from build123d import *

# Parameters (mm, degrees)
F1_DEPTH = 34.925
F2_DEPTH = 11.1125
F3_SIZE2 = 11.11249
F3_SIZE  = 4.602938


# Not quite as in the source:
# - a fillet or chamfer is up to 0.001 mm smaller than in the source, because OpenCascade refuses the exact size


with BuildPart() as f1:
    # F0 (on Top) → F1 (new body)
    with BuildSketch(Plane.XY):
        Polygon((0, -134.14375), (0, 134.14375), (-73.81875, 0), align=None)
        Polygon((73.81875, 0), (0, 134.14375), (0, -134.14375), align=None)
    extrude(amount=-F1_DEPTH)

    # F0 (on Top) + F1_face (on face) → F2 (join)
    with BuildSketch(Plane.XY):
        Polygon((-103.1875, 0), (0, -187.5127688172), (103.1875, 0), (0, 187.5127688172), align=None)
        Polygon((-73.81875, 0), (0, 134.14375), (73.81875, 0), (0, -134.14375), align=None, mode=Mode.SUBTRACT)
    with BuildSketch(Plane.XY):
        Polygon((0, 134.14375), (-73.81875, 0), (0, -134.14375), (73.81875, 0), align=None)
    extrude(amount=F2_DEPTH)

    # F3 (size 4.6029482119 and 11.1125 in the source; OpenCascade refuses exactly that, so slightly less here)
    f3_edges = [f1.edges().sort_by_distance(p)[0] for p in [
        (-51.59375, -93.756384, 11.1125),
        (-51.59375, 93.756384, 11.1125),
        (51.59375, 93.756384, 11.1125),
        (51.59375, -93.756384, 11.1125),
    ]]
    f3_side = f1.faces().sort_by_distance((0, 0, 11.1125))[0]
    chamfer(f3_edges, length=F3_SIZE, length2=F3_SIZE2, reference=f3_side)


solid = f1.part
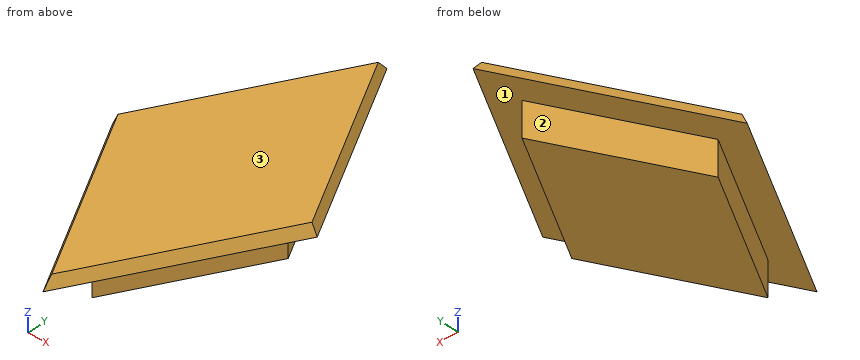
Input: part model. Units: mm. Frame: model coordinates. Face numbers are marked on the shaded views. A direction names the side the tool comes from. Give positions to 0.01 mm unless a question says otherwise; leave off trailing zeros. Order: outer loops, then holes, each group sorted by start corner. A loop starts at its lowest first (then second) coordinate and runs counter-clockwise, first axis right, second up.
Q1. Section C-C on z = -16. Output: boundary loops of the cut face in (x, y).
Checked values:
outline: (-73.82, 0) - (0, -134.14) - (73.82, 0) - (0, 134.14) - close
Q2. Ray query, probe 1 along X at (y, z) = (-92.5, 2.5); probe 2 along Y at (x, z) = (28, -25.5); probe 3 along X at (y, z) = (101.5, -11). Return the intervals inside material, ascending.
Checked values:
probe 1: x = -51.1 to 51.1
probe 2: y = -83.26 to 83.26
probe 3: x = -17.96 to 17.96
Q3. Contact query for flat-ended pins moving along their axis: pin 1 Ø10 at (x, z) = (73, -13) entering from +Y; pin 2 Ø5 at (x, z) = (23, -24) entering from -Y; pin 3 Ø8 at (x, y) = (63.5, -81) entering from -Z; pin 4 Ø1 at (y, z) = (85, 6.5) entering from -X. Output: stop coordinate, or through.
Checked values:
pin 1: stops at y = 10.57
pin 2: stops at y = -96.89
pin 3: passes through
pin 4: stops at x = -53.7
Q4. Set-up query: the marked faces 1, 2 and 3. Return all of +Z, -Z, +X, -X, +Y, -Y with unobstructed straight access to the full face (end or side cutting, diameter ignored); none if empty.
Checked values:
face 1: -Z
face 2: -Z, -X, +Y
face 3: +Z, +X, -X, +Y, -Y
